from build123d import *

# Parameters (mm, degrees)
SKETCH_1_W          = 24
SKETCH_1_H          = 36
EXTRUDE_1_DEPTH     = 2
FILLET_1_R          = 2
SKETCH_4_R          = 2.05
CUT_EXTRUDE_1_DEPTH = 1
SKETCH_7_R          = 4.75
SKETCH_7_R_2        = 4
EXTRUDE_2_DEPTH     = 4
CUT_EXTRUDE_2_DEPTH = 4
SKETCH_9_R          = 1
CUT_EXTRUDE_3_DEPTH = 1
CUT_EXTRUDE_4_REACH = 146.567
SKETCH_10_R         = 0.5
EXTRUDE_3_DEPTH     = 4


with BuildPart() as part:
    # 草图1 → 凸台-拉伸1 (new body)
    with BuildSketch(Plane.XY):
        with Locations((-109.790086771, 59.72858385)):
            Rectangle(SKETCH_1_W, SKETCH_1_H)
    extrude(amount=EXTRUDE_1_DEPTH)

    # 圆角1
    fillet_1_edges = [part.edges().sort_by_distance(p)[0] for p in [
        (-121.790086771, 59.72858385, 2),
        (-109.790086771, 41.72858385, 2),
        (-97.790086771, 59.72858385, 2),
        (-97.790086771, 41.72858385, 1),
        (-121.790086771, 41.72858385, 1),
        (-121.790086771, 77.72858385, 1),
        (-97.790086771, 77.72858385, 1),
        (-109.790086771, 77.72858385, 2),
    ]]
    fillet(fillet_1_edges, radius=FILLET_1_R - 0.0001)  # a hair under: the kernel refuses the full size

    # 草图4 → 切除-拉伸1 (cut)
    with BuildSketch(Plane(origin=(0, 0, 0), x_dir=(-1, 0, 0), z_dir=(0, 0, -1))):
        with Locations((117.420086771, 66.20858385)):
            Circle(SKETCH_4_R)
    extrude(amount=-CUT_EXTRUDE_1_DEPTH, mode=Mode.SUBTRACT)

    # 草图7 → 凸台-拉伸2 (add)
    with BuildSketch(Plane(origin=(0, 0, 0), x_dir=(-1, 0, 0), z_dir=(0, 0, -1))):
        with Locations((105.790086771, 70.72858385)):
            Circle(SKETCH_7_R)
        with Locations((105.790086771, 70.72858385)):
            Circle(SKETCH_7_R_2, mode=Mode.SUBTRACT)
    extrude(amount=EXTRUDE_2_DEPTH)

    # 草图8 → 切除-拉伸2 (cut)
    with BuildSketch(Plane(origin=(0, 0, -4), x_dir=(-1, 0, 0), z_dir=(0, 0, -1))):
        Polygon((107.295042198, 64.806439923), (104.296751001, 64.705198151), (104.296751001, 67.705198151), (107.295042198, 67.705198151), align=None)
    extrude(amount=-CUT_EXTRUDE_2_DEPTH, mode=Mode.SUBTRACT)

    # 草图9 → 切除-拉伸3 (cut)
    with BuildSketch(Plane.XY.offset(2)):
        with Locations((-100.790086771, 74.72858385)):
            Circle(SKETCH_9_R)
        with Locations((-100.790086771, 44.72858385)):
            Circle(SKETCH_9_R)
        with Locations((-118.790086771, 44.72858385)):
            Circle(SKETCH_9_R)
        with Locations((-118.790086771, 74.72858385)):
            Circle(SKETCH_9_R)
    extrude(amount=-CUT_EXTRUDE_3_DEPTH, mode=Mode.SUBTRACT)

    # 草图10 → 切除-拉伸4 (cut, up to next)
    with BuildSketch(Plane.XY.offset(1), mode=Mode.PRIVATE) as cut_extrude_4_sk1:
        with Locations((-118.790086771, 44.72858385)):
            Circle(SKETCH_10_R)
    cut_extrude_4_tool1 = extrude(cut_extrude_4_sk1.sketch, amount=-CUT_EXTRUDE_4_REACH, mode=Mode.PRIVATE) & part.part
    # 草图10 → 切除-拉伸4 (cut, up to next)
    with BuildSketch(Plane.XY.offset(1), mode=Mode.PRIVATE) as cut_extrude_4_sk2:
        with Locations((-100.790086771, 44.72858385)):
            Circle(SKETCH_10_R)
    cut_extrude_4_tool2 = extrude(cut_extrude_4_sk2.sketch, amount=-CUT_EXTRUDE_4_REACH, mode=Mode.PRIVATE) & part.part
    # 草图10 → 切除-拉伸4 (cut, up to next)
    with BuildSketch(Plane.XY.offset(1), mode=Mode.PRIVATE) as cut_extrude_4_sk3:
        with Locations((-100.790086771, 74.72858385)):
            Circle(SKETCH_10_R)
    cut_extrude_4_tool3 = extrude(cut_extrude_4_sk3.sketch, amount=-CUT_EXTRUDE_4_REACH, mode=Mode.PRIVATE) & part.part
    # 草图10 → 切除-拉伸4 (cut, up to next)
    with BuildSketch(Plane.XY.offset(1), mode=Mode.PRIVATE) as cut_extrude_4_sk4:
        with Locations((-118.790086771, 74.72858385)):
            Circle(SKETCH_10_R)
    cut_extrude_4_tool4 = extrude(cut_extrude_4_sk4.sketch, amount=-CUT_EXTRUDE_4_REACH, mode=Mode.PRIVATE) & part.part
    add(cut_extrude_4_tool1.solids().sort_by_distance((-118.790087, 44.728584, 1))[0], mode=Mode.SUBTRACT)
    add(cut_extrude_4_tool2.solids().sort_by_distance((-100.790087, 44.728584, 1))[0], mode=Mode.SUBTRACT)
    add(cut_extrude_4_tool3.solids().sort_by_distance((-100.790087, 74.728584, 1))[0], mode=Mode.SUBTRACT)
    add(cut_extrude_4_tool4.solids().sort_by_distance((-118.790087, 74.728584, 1))[0], mode=Mode.SUBTRACT)

    # 草图12 → 凸台-拉伸3 (add)
    with BuildSketch(Plane(origin=(0, 0, 0), x_dir=(-1, 0, 0), z_dir=(0, 0, -1))):
        with BuildLine():
            Line((108.145924466, 66.861652665), (111.46923478, 59.734790696))
            ThreePointArc((111.46923478, 59.734790696), (111.253339507, 59.141623309), (110.66017212, 59.357518582))
            Line((110.66017212, 59.357518582), (107.336861805, 66.484380551))
            ThreePointArc((107.336861805, 66.484380551), (107.552757078, 67.077547938), (108.145924466, 66.861652665))
        make_face()
    extrude(amount=EXTRUDE_3_DEPTH)


solid = part.part
For this review, take the finished solid that the model builds, in its own axes (mm). A direction names the side the tool comes from. Coordinates: 2 decimals unless noted, no trailing zeros. Write each loop counter-clockwise with the first axis right and the second up, starting at its lowest first coordinate (ties: lowest second). Pieces come first, ordered by that corner, then holes. Notation, with made-up numbers: (-10.75, 55) -> (27.25, 55) arc R19 ccw to (27.25, 81) -> close; hole circle Ø6 at (-7.75, 32). An arc over 180 degrees is marked (long way). Write each question's results on one line, items separated by ' | '. Start each with the question number.
1) The part is to be moulded in two halves that separate along X. For faces 4 (the face through (-101, 44, 1)), 5 (the face through (-110, 60, 2)), 6 (the face through (-105.443, 75.466, -1.972)), say which applies: +X half, -X half, draft (parallel to the pull), parting line (faces both ways), or undercut.
2) Consider section A-A (z = 0.45). Write out the cut boundary in (x, y), plus the area to 3 significant figures.
3) Insertion check: pin 1 (1 mm diameter, centred on x = -101, y = 44.5, fed in from +Z); pin 2 (13 mm diameter, centred on x = -105.79, y = 70.73, fed in from -Z); pin 3 (1.5 mm diameter, centred on x = -106, z = 1, fed in from -Y); pin 4 (1.6 mm diameter, centred on x = -118.79, y = 44.73, fed in from -Z). Each pin has a flat end and moves straight along its axis. Give the tip position at first contact, or say it passes through.
4) Wall thickness on L1, parallel to Z at x = -118.75, y = 54; L2, parallel to Z at x = -118.25, y = 75.5; L3, parallel to X at y = 68.5, z = -0.3: over which ranges is each line inside the solid? List them lowest first. Write a range as [from, to].
5) For faces 1 (the face through (-117, 66, 1)), 2 (the face through (-100.328, 44.537, 0.507)), 3 (the face through (-100, 75, 1)), list the 3-axis set-ups (+Z, -Z, +X, -X, +Y, -Y) from which the entire face can be reached by the end or side of a thin tool; tool diameter is ignored.
6) Consider section D-D (z = -1.55). Write out the cut boundary in (x, y).
Geometry says:
1) face 4: undercut | face 5: draft | face 6: parting line
2) outline: (-121.74, 43.73) arc R1.95 ccw to (-119.79, 41.78) -> (-99.79, 41.78) arc R1.95 ccw to (-97.84, 43.73) -> (-97.84, 75.73) arc R1.95 ccw to (-99.79, 77.68) -> (-119.79, 77.68) arc R1.95 ccw to (-121.74, 75.73) -> close; hole circle Ø4.1 at (-117.42, 66.21); hole circle Ø1 at (-118.79, 44.73); hole circle Ø1 at (-118.79, 74.73); hole circle Ø1 at (-100.79, 44.73); hole circle Ø1 at (-100.79, 74.73) | area: 838 mm^2
3) pin 1: z = 1 | pin 2: z = -4 | pin 3: y = 41.74 | pin 4: z = 0
4) L1: [0, 2] | L2: [0, 1] | L3: [-109.98, -109.11], [-102.47, -101.6]
5) face 1: -Z | face 2: +Z, -Z | face 3: +Z
6) outline: (-111.47, 59.73) arc R0.45 ccw to (-110.66, 59.36) -> (-107.44, 66.27) arc R4.75 ccw to (-107.3, 66.22) -> (-107.3, 67.02) arc R4 cw (long way) to (-104.3, 67.02) -> (-104.3, 66.22) arc R4.75 ccw (long way) to (-108.24, 66.66) -> close
